Geometry check sheet. Reference: the model listing, model coordinates, mm. Round coordinates to 2 decimals unless told otherwise and drop trailing zeros. Write each loop counter-clockwise with the first axis right and the second up, starting at its lowest first coordinate (ties: lowest second). Pieces come first, ordered by that corner, then holes. Notation, with made-up numbers: (75, -24) - (97, -24) arc R4 ccw to (97, -17) - close; hole circle Ø9 at (32.25, 77.25). An arc over 180 degrees is marked (long way). Return JSON: item names as keys, results as strings. Group by question number.
Solid Edge part; units mm, degrees
sketch "Sketch1" plane through (0, 0, 0) normal (0, 0, 1) x (1, 0, 0)
  line L0 (12.5, 7.5) -> (-10, 7.5)
  line L1 (-10, 7.5) -> (-10, -7.5)
  line L2 (-10, -7.5) -> (12.5, -7.5)
  line L3 (12.5, -7.5) -> (12.5, 7.5)
extrude "Protrusion1" add sketch "Sketch1" along normal blind 1
fillet "Round_1" radius 0.5 4 edges at (12.5, 7.5, 0.5) (12.5, -7.5, 0.5) (-10, -7.5, 0.5) (-10, 7.5, 0.5)
hole "Hole_1" at (-2.5, 0, 1) direction (0, 0, -1) diameter 3 end up to next
hole "Hole_2" at (-8, 5, 1) direction (0, 0, -1) diameter 1.5 end up to next
hole "Hole1" at (-8, 3, 1) direction (0, 0, -1) diameter 1.5 end up to next
hole "Hole2" at (-8, 1, 1) direction (0, 0, -1) diameter 1.5 end up to next
hole "Hole3" at (-8, -1, 1) direction (0, 0, -1) diameter 1.5 end up to next
hole "Hole4" at (-8, -3, 1) direction (0, 0, -1) diameter 1.5 end up to next
hole "Hole5" at (-8, -5, 1) direction (0, 0, -1) diameter 1.5 end up to next
1. Section check C-C (y = 3). Enter the section's corners in (x, z), and give its area (3 significant figures).
2. Material ranges on line 1 along X through (y, z) = (-3, 0.8); line 2 along X through (y, z) = (-1, 0.4); line 3 along X through (y, z) = (0, 0.2), recorded low to high.
3. Section check D-D (x = -8). Enter the section's corners in (y, z).
4. Section check B-B (z = 0.55). Enter the section's corners in (x, y).
5. Section check A-A (x = -2.5). Enter the section's corners in (y, z).
6. Mould release check, pull along Y, two halves, no side actions. Record for faces 1 (the face through (1.1, -7.5, 0.5)), 2 (the face through (-10, 0.1, 0.5)), 3 (the face through (-7.775, 0.285, 0.507)), 4 (the face through (1.4, 7.5, 0.5)): pulls with the +Y half, pulls with the -Y half, needs draft (parallel to the pull), parting line crosses it, or undercut.
7. Depth check by flat-ended pin: pin 1 Ø1.5 at (x, y) = (5, -4) entering from -Z. Enter the tip coordinate at first touch or a pass-through.
Result sheet:
{
 "1": {"outline": "(-10, 0) - (-8.75, 0) - (-8.75, 1) - (-10, 1) - close; (-7.25, 0) - (12.5, 0) - (12.5, 1) - (-7.25, 1) - close", "area": "21.0 mm²"},
 "2": {"line 1": "x = -10 to -8.75, -7.25 to 12.5", "line 2": "x = -10 to -8.75, -7.25 to -3.62, -1.38 to 12.5", "line 3": "x = -10 to -4, -1 to 12.5"},
 "3": {"outline": "(-7.5, 0) - (-5.75, 0) - (-5.75, 1) - (-7.5, 1) - close; (-4.25, 0) - (-3.75, 0) - (-3.75, 1) - (-4.25, 1) - close; (-2.25, 0) - (-1.75, 0) - (-1.75, 1) - (-2.25, 1) - close; (-0.25, 0) - (0.25, 0) - (0.25, 1) - (-0.25, 1) - close; (1.75, 0) - (2.25, 0) - (2.25, 1) - (1.75, 1) - close; (3.75, 0) - (4.25, 0) - (4.25, 1) - (3.75, 1) - close; (5.75, 0) - (7.5, 0) - (7.5, 1) - (5.75, 1) - close"},
 "4": {"outline": "(-10, -7) arc R0.5 ccw to (-9.5, -7.5) - (12, -7.5) arc R0.5 ccw to (12.5, -7) - (12.5, 7) arc R0.5 ccw to (12, 7.5) - (-9.5, 7.5) arc R0.5 ccw to (-10, 7) - close; hole circle Ø1.5 at (-8, -5); hole circle Ø1.5 at (-8, -3); hole circle Ø1.5 at (-8, -1); hole circle Ø1.5 at (-8, 1); hole circle Ø1.5 at (-8, 3); hole circle Ø1.5 at (-8, 5); hole circle Ø3 at (-2.5, 0)"},
 "5": {"outline": "(-7.5, 0) - (-1.5, 0) - (-1.5, 1) - (-7.5, 1) - close; (1.5, 0) - (7.5, 0) - (7.5, 1) - (1.5, 1) - close"},
 "6": {"face 1": "pulls with the -Y half", "face 2": "needs draft", "face 3": "undercut", "face 4": "pulls with the +Y half"},
 "7": {"pin 1": "stops at z = 0"}
}
